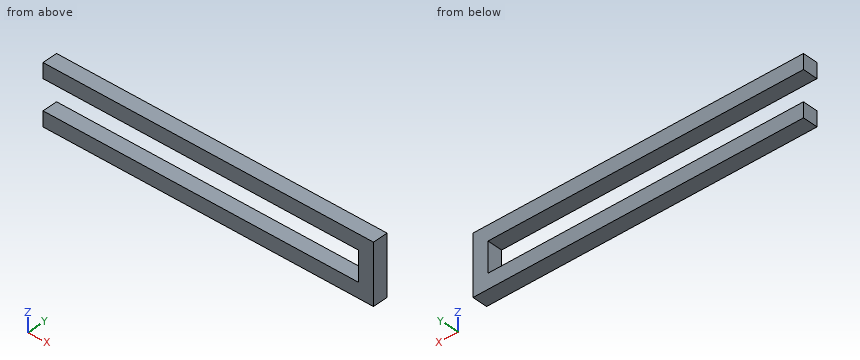
```python
from build123d import *

# Parameters (mm, degrees)
SKETCH1_W           = 210
SKETCH1_H           = 10
BOSS_EXTRUDE1_DEPTH = 10


with BuildPart() as part:
    # Sketch1 → Boss-Extrude1 (new body)
    with BuildSketch(Plane(origin=(0, 0, 0), x_dir=(1, 0, 0), z_dir=(0, 1, 0))):
        with Locations((77.998094374, -14.015426497)):
            Rectangle(SKETCH1_W, SKETCH1_H)
        Polygon((192.998094374, 20.984573503), (182.998094374, 20.984573503), (182.998094374, 10.984573503), (182.998094374, -9.015426497), (182.998094374, -19.015426497), (192.998094374, -19.015426497), align=None)
        with Locations((77.998094374, 15.984573503)):
            Rectangle(SKETCH1_W, SKETCH1_H)
    extrude(amount=BOSS_EXTRUDE1_DEPTH)


solid = part.part
```
For this review, take the finished solid that the model builds, in its own axes (mm). Coordinates: 2 decimals unless noted, no trailing zeros. Loops run counter-clockwise (first coordinate to the right, second up) from the corner with the lowest first, then second, coordinate; pieces in that order, holes last. Notation, with made-up numbers: (79, 30) - (95, 30) arc R33 cw to (95, 63) - close; hole circle Ø9 at (-13.75, -34.75). An arc over 180 degrees is marked (long way). Use one line per item in the form item = value. Start each with the question number.
1) For pin 1 (5 mm diameter, centred on y = 5, z = -1.5, fed in from -X), flat-tipped, find the tip position at first contact; note if it passes through.
2) Take a section at B-B (y = 1.5). State the section outline as (x, z) points.
3) To check wall thickness, follow probe 1 along Z at (x, y) = (16, 2); probe 2 along X at (y, z) = (8.5, 0). State the ranges of each line that lie inside material, in increasing order. Write a range as from..to.
4) Take a section at C-C (z = -6). State the section outline as (x, y) points.
5) Take a section at A-A (x = 131.5). State the section outline as (y, z) points, plus the area to 3 significant figures.
From the geometry:
q1.pin_1 = 183
q2.outline = (-27, -20.98) - (193, -20.98) - (193, 19.02) - (-27, 19.02) - (-27, 9.02) - (183, 9.02) - (183, -10.98) - (-27, -10.98) - close
q3.probe_1 = -20.98..-10.98, 9.02..19.02
q3.probe_2 = 183..193
q4.outline = (183, 0) - (193, 0) - (193, 10) - (183, 10) - close
q5.outline = (0, -20.98) - (10, -20.98) - (10, -10.98) - (0, -10.98) - close; (0, 9.02) - (10, 9.02) - (10, 19.02) - (0, 19.02) - close
q5.area = 200 mm2
